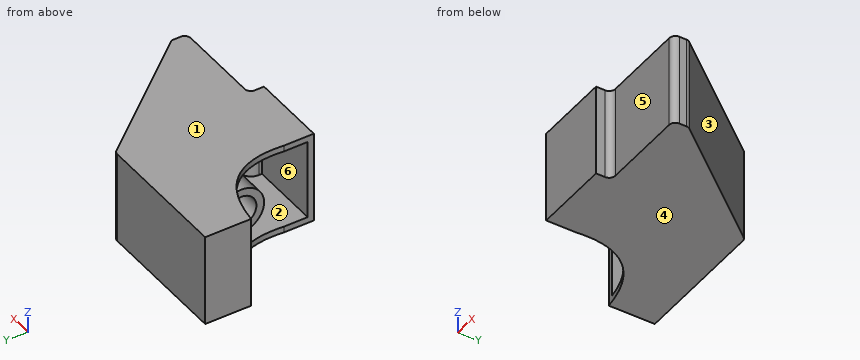
```python
from build123d import *

# Parameters (mm, degrees)
BOSS_EXTRUDE1_DEPTH             = 38.1
SHELL1_START                    = 2.54
SHELL1_DEPTH                    = 33.02
SKETCH2_R                       = 9.525
SKETCH2_R_2                     = 6.35
BOSS_EXTRUDE2_DEPTH             = 35.56
BOSS_EXTRUDE2_DIRECTION_2_REACH = 98.336


# Read off the part's stored shape, not the designer's step: Shell1
with BuildPart() as part:
    # Sketch1 → Boss-Extrude1 (new body)
    with BuildSketch(Plane.XY):
        with BuildLine():
            Line((-28.597743471, 0), (27.367835077, 0))
            ThreePointArc((27.367835077, 0), (28.441285462, -0.237978221), (29.313587963, -0.907319471))
            Line((29.313587963, -0.907319471), (70.584270678, -50.091803866))
            ThreePointArc((70.584270678, -50.091803866), (71.025337049, -50.855753231), (71.178517793, -51.724484395))
            Line((71.178517793, -51.724484395), (71.178517793, -54.61))
            ThreePointArc((71.178517793, -54.61), (70.434569017, -56.406051224), (68.638517793, -57.15))
            Line((68.638517793, -57.15), (34.29, -57.15))
            ThreePointArc((34.29, -57.15), (32.493948776, -57.893948776), (31.75, -59.69))
            Line((31.75, -59.69), (31.75, -63.5))
            Line((31.75, -63.5), (0, -63.5))
            Line((0, -63.5), (0, -51.225562477))
            add(Edge.make_bspline(
                [(-28.597743471, -19.05), (2.699862554, -22.282217033), (0, -51.225562477)],
                knots=[0, 0, 0, 1, 1, 1], degree=2))
            Line((-28.597743471, -19.05), (-28.597743471, 0))
        make_face()
    extrude(amount=BOSS_EXTRUDE1_DEPTH)

    # Shell1 outline → Shell1 (cut)
    with BuildSketch(Plane.XY.offset(SHELL1_START)):
        with BuildLine():
            Line((-26.057743471, -2.54), (-26.057743471, -19.362677405))
            add(Edge.make_bspline(
                [(-26.057743471, -19.362677405), (2.587779826, -23.483777864), (0, -51.225562477)],
                knots=[0.041514235, 0.041514235, 0.041514235, 1, 1, 1], degree=2))
            Line((0, -51.225562477), (0, -60.96))
            Line((0, -60.96), (29.21, -60.96))
            Line((29.21, -60.96), (29.21, -59.69))
            ThreePointArc((29.21, -59.69), (30.697897552, -56.097897552), (34.29, -54.61))
            Line((34.29, -54.61), (68.638517793, -54.61))
            Line((68.638517793, -54.61), (68.638517793, -51.724484395))
            Line((68.638517793, -51.724484395), (27.367835077, -2.54))
            Line((27.367835077, -2.54), (-26.057743471, -2.54))
        make_face()
    extrude(amount=SHELL1_DEPTH, mode=Mode.SUBTRACT)

    # Sketch2 → Boss-Extrude2 (add)
    with BuildSketch(Plane.ZY.offset(-33.02)):
        with Locations((19.05, -31.75)):
            Circle(SKETCH2_R)
        with Locations((19.05, -31.75)):
            Circle(SKETCH2_R_2, mode=Mode.SUBTRACT)
    extrude(amount=BOSS_EXTRUDE2_DEPTH)

    # Boss-Extrude2 direction 2: up to this face of the body (flat: up to its plane)
    boss_extrude2_direction_2_end = Plane(part.part.faces().sort_by_distance((48.003176435, -27.132242197, 19.05))[0])
    # Sketch2 → Boss-Extrude2 direction 2 (add, up to the picked face)
    with BuildSketch(Plane.ZY.offset(-33.02), mode=Mode.PRIVATE) as boss_extrude2_direction_2_sk1:
        with Locations((19.05, -31.75)):
            Circle(SKETCH2_R)
        with Locations((19.05, -31.75)):
            Circle(SKETCH2_R_2, mode=Mode.SUBTRACT)
    boss_extrude2_direction_2_tool1 = split(extrude(boss_extrude2_direction_2_sk1.sketch, amount=-BOSS_EXTRUDE2_DIRECTION_2_REACH, mode=Mode.PRIVATE), bisect_by=boss_extrude2_direction_2_end, keep=Keep.BOTH, mode=Mode.PRIVATE)
    add(boss_extrude2_direction_2_tool1.solids().sort_by(Axis((33.02, -31.75, 9.794408), (1, 0, 0)))[0])


solid = part.part
```
Input: part model. Units: mm. Frame: model coordinates. Face numbers are marked on the shaded views. A direction names the side the tool comes from. Give positions to 0.01 mm unless a question says otherwise; leave off trailing zeros. Order: outer loops, then holes, each group sorted by start corner. A loop starts at its lowest first (then second) coordinate and runs counter-clockwise, first axis right, second up. Notation, with made-up numbers: (52.5, 19.25) - (107.5, 19.25) arc R26 cw to (107.5, 47.25) - close; hole circle Ø8 at (68, 73). An arc over 180 degrees is marked (long way). One line per item, written item: value.
1. Cut plane B-B, the plane y = -18. Output: boundary loops of the cut face in (x, z), and give its area (3 significant figures).
Determined:
outline: (-28.6, 0) - (43.66, 0) - (43.66, 38.1) - (-28.6, 38.1) - close; hole (-26.06, 2.54) - (40.34, 2.54) - (40.34, 35.56) - (-26.06, 35.56) - close
area: 560 mm2
2. Reachability of the marked faces 4, 5 and 6 from +Z, -Z, +X, -X, +Y, -Y: full face, straight path, thin tool, end or side. Return the list, or none.
Determined:
face 4: -Z, +X, -X, +Y, -Y
face 5: +Z, -Z, +X, -Y
face 6: -X
3. Line query: probe 1 along Y at (x, z) = (15.5, 19.05) (3 decimals); probe 2 along Z at (x, y) = (17, -31); probe 3 along Z at (x, y) = (57.5, -45). Output: solid intervals per line, ascending.
Determined:
probe 1: -63.5 to -60.96, -41.275 to -38.1, -25.4 to -22.225, -2.54 to 0
probe 2: 0 to 2.54, 9.55 to 12.74, 25.36 to 28.55, 35.56 to 38.1
probe 3: 0 to 2.54, 35.56 to 38.1
4. Cut plane C-C, the plane y = -56. Output: boundary loops of the cut face in (x, z).
Determined:
outline: (0, 0) - (70.76, 0) - (70.76, 38.1) - (0, 38.1) - (0, 35.56) - (30.8, 35.56) - (30.8, 2.54) - (0, 2.54) - close
5. Cut plane A-A, the plane x = 13.5. Output: boundary loops of the cut face in (y, z) (3 decimals).
Determined:
outline: (-63.5, 0) - (0, 0) - (0, 38.1) - (-63.5, 38.1) - close; circle Ø19.05 at (-31.75, 19.05); hole (-60.96, 2.54) - (-2.54, 2.54) - (-2.54, 35.56) - (-60.96, 35.56) - close; hole circle Ø12.7 at (-31.75, 19.05)
6. Draft query along X for the marked faces 1, 2 and 3. Return one class per face: released by +X, released by -X, zero draft, split by the parting line, or undercut.
Determined:
face 1: zero draft
face 2: undercut
face 3: released by +X
7. Pin query (flat end, axial travel): pin 1 Ø3 at (y, z) = (-53.5, 13.5) entering from -X; pin 2 Ø10 at (y, z) = (-31.75, 19.05) entering from -X; pin 3 Ø4 at (y, z) = (-62.5, 24) entering from +X. Return the tip coordinate at first contact, or that it passes through.
Determined:
pin 1: x = 32.34
pin 2: x = 47.68
pin 3: x = 31.75
